Geometry: final body of the model. Coordinates: model frame, mm. A direction names the side the tool comes from. Give positions to 0.01 mm unless a question says otherwise; leave off trailing zeros. Write each loop counter-clockwise with the first axis right and the second up, starting at its lowest first coordinate (ties: lowest second). Pieces come first, ordered by that corner, then holes.
from build123d import *

# Parameters (mm, degrees)
BOSS_EXTRUDE2_DEPTH = 25.4
FILLET1_R           = 12.7
FILLET2_R           = 12.7


with BuildPart() as part:
    # Sketch3 → Boss-Extrude2 (new body)
    with BuildSketch(Plane.XY):
        with BuildLine():
            Line((-177.8, 7.57860608), (-177.8, -129.54))
            Line((-177.8, -129.54), (-182.88, -129.54))
            Line((-182.88, -129.54), (-182.88, 7.57860608))
            add(Edge.make_bspline(
                [(182.88, 7.57860608), (182.88, 46.763821962), (0, 141.394473708), (-182.88, 58.90806056), (-182.88, 7.57860608)],
                knots=[0, 0, 0, 0, 0.5, 1, 1, 1, 1], degree=3))
            Line((182.88, 7.57860608), (182.88, -129.54))
            Line((182.88, -129.54), (177.8, -129.54))
            Line((177.8, -129.54), (177.8, 7.57860608))
            add(Edge.make_bspline(
                [(-177.8, 7.57860608), (-177.8, 46.300078228), (0, 128.042210108), (177.8, 30.017127825), (177.8, 7.57860608)],
                knots=[0, 0, 0, 0, 0.5, 1, 1, 1, 1], degree=3))
        make_face()
    extrude(amount=BOSS_EXTRUDE2_DEPTH)

    # Fillet1
    fillet1_edges = [part.edges().sort_by_distance(p)[0] for p in [
        (-180.34, -129.54, 0),
        (-180.34, -129.54, 25.4),
    ]]
    fillet(fillet1_edges, radius=FILLET1_R - 0.0001)  # a hair under: the kernel refuses the full size

    # Fillet2
    fillet2_edges = [part.edges().sort_by_distance(p)[0] for p in [
        (180.34, -129.54, 0),
        (180.34, -129.54, 25.4),
    ]]
    fillet(fillet2_edges, radius=FILLET2_R - 0.0001)  # a hair under: the kernel refuses the full size


solid = part.part
Q1. Pin query (flat end, axial travel): P1, Ø1, axis at x = 85, z = 6, coming from the -Y side; P2, Ø5, axis at y = 37, z = 17, coming from the +X side. Return the tip coordinate at first contact, or that it passes through.
Filled sheet:
P1: stops at y = 66.73
P2: stops at x = 170.18
Q2. Ray query, line 1 along X through (y, z) = (-59, 2.5); line 2 along Y through (x, z) = (-71.5, 1.25); line 3 along Y through (x, z) = (93.5, 7.75). Return the intervals inside material, ascending.
Filled sheet:
line 1: x = -182.88 to -177.8, 177.8 to 182.88
line 2: y = 77.24 to 90.73
line 3: y = 63.99 to 79.41
Q3. Access query for faces 4 (the flat face through (177.8, -62, 13)), 5 (the cylindrical face through (-180.4, -125.9, 3.8)). Directions: +Z, -Z, +X, -X, +Y, -Y. A direction counts if a zero-diameter tool reaches every point of the face in a straight line with its end or side. Return the directions, or none.
Filled sheet:
face 4: +Z, -Z, -Y
face 5: -Z, +X, -X, -Y
Q4. Section A-A on y = -104. Output: boundary loops of the cut face in (x, z).
Filled sheet:
outline: (-182.88, 0) - (-177.8, 0) - (-177.8, 25.4) - (-182.88, 25.4) - close; (177.8, 0) - (182.88, 0) - (182.88, 25.4) - (177.8, 25.4) - close
Q5. Pull-direction query (X, two-part tool) for faces 1 (the cylindrical face through (180.3, -125.7, 21.8)), 2 (the flat face through (182.88, -60, 13)), 3 (the flat face through (-177.8, -60, 13)); classes: released by +X, released by -X, zero draft, split by the parting line, or undercut.
Filled sheet:
face 1: zero draft
face 2: released by +X
face 3: undercut
